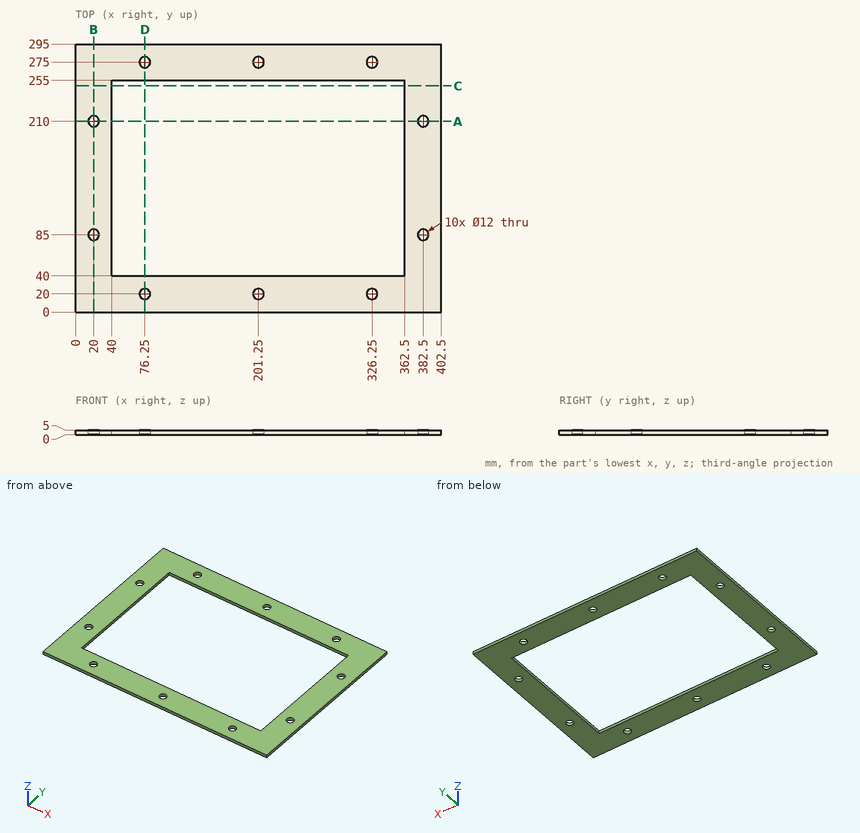
Here's the drawing with two shaded views (mm, measured from the low corner). I have some questions. Give positions to 0.01 mm unless a question says otherwise; leave off trailing zeros. Write each loop counter-clockwise with the first axis right and the second up, starting at its lowest first coordinate (ties: lowest second). Pieces come first, ordered by that corner, then holes. Notation, with made-up numbers: (2.5, -38) - (30.5, -38) arc R25 cw to (30.5, -3) - close; hole circle Ø8 at (-10, 83.5). An arc over 180 degrees is marked (long way). Write item = value, one per line. Start each with the question number.
1. Imagine slicing it at D-D (x = 76.25). Please give me the cut outline in (y, z), and give its area (3 significant figures).
2. Imagine slicing it at A-A (y = 210). Please give me the cut outline in (x, z), and give its area (3 significant figures).
3. Imagine slicing it at B-B (x = 20). Please give me the cut outline in (y, z).
4. For pin 1 (7 mm diameter, centred on x = 20, y = 85, fed in from -Z), with a flat end and sliding along its axis, tell me the tip position at first contact or that it passes through.
5. Imagine slicing it at C-C (y = 249). Please give me the cut outline in (x, z).
6. Please list where these lines run through material, in increasing order: line 1 (Y direction, x = 382.5, z = 1.5); line 2 (Y direction, x = 201.25, z = 3.55); line 3 (X direction, y = 20, z = 2.25).
Worked answers:
q1.outline = (0, 0) - (14, 0) - (14, 5) - (0, 5) - close; (26, 0) - (40, 0) - (40, 5) - (26, 5) - close; (255, 0) - (269, 0) - (269, 5) - (255, 5) - close; (281, 0) - (295, 0) - (295, 5) - (281, 5) - close
q1.area = 280 mm2
q2.outline = (0, 0) - (14, 0) - (14, 5) - (0, 5) - close; (26, 0) - (40, 0) - (40, 5) - (26, 5) - close; (362.5, 0) - (376.5, 0) - (376.5, 5) - (362.5, 5) - close; (388.5, 0) - (402.5, 0) - (402.5, 5) - (388.5, 5) - close
q2.area = 280 mm2
q3.outline = (0, 0) - (79, 0) - (79, 5) - (0, 5) - close; (91, 0) - (204, 0) - (204, 5) - (91, 5) - close; (216, 0) - (295, 0) - (295, 5) - (216, 5) - close
q4.pin_1 = through
q5.outline = (0, 0) - (40, 0) - (40, 5) - (0, 5) - close; (362.5, 0) - (402.5, 0) - (402.5, 5) - (362.5, 5) - close
q6.line_1 = 0 to 79, 91 to 204, 216 to 295
q6.line_2 = 0 to 14, 26 to 40, 255 to 269, 281 to 295
q6.line_3 = 0 to 70.25, 82.25 to 195.25, 207.25 to 320.25, 332.25 to 402.5
